For this review, take the finished solid that the model builds, in its own axes (mm). Face numbers are marked on the shaded views. A direction names the side the tool comes from. Coordinates: 2 decimals unless noted, no trailing zeros. Order: outer loops, then holes, each group sorted by start corner. A loop starts at its lowest first (then second) coordinate and runs counter-clockwise, first axis right, second up. Notation, with made-up numbers: M 10.25,-15 L 25.25,-15 A36 ccw 25.25,22 Z; hole C 47.25,-31 d1. An arc over 180 degrees is marked long. Use one line per item in the form item = value. Start each with the question number.
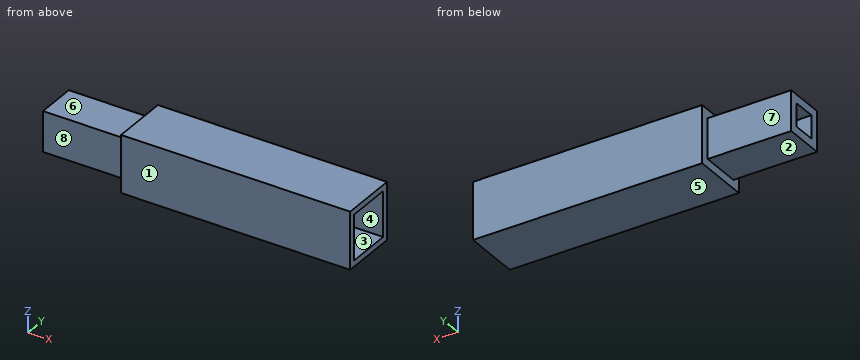
Autodesk Inventor part; units mm, degrees
ref_plane "YZ Plane" through (0, 0, 0) normal (1, 0, 0) x (0, 1, 0)
ref_plane "XZ Plane" through (0, 0, 0) normal (0, 1, 0) x (-1, 0, 0)
ref_plane "XY Plane" through (0, 0, 0) normal (0, 0, 1) x (1, 0, 0)
sketch "Sketch1" plane through (0, 0, 0) normal (1, 0, 0) x (0, 1, 0)
  line L0 (0, 0) -> (25.4, 0)
  line L1 (25.4, 0) -> (25.4, -25.4)
  line L2 (25.4, -25.4) -> (0, -25.4)
  line L3 (0, -25.4) -> (0, 0)
  line L4 (0, 0) -> (3.175, 0)
  line L5 (0, -3.175) -> (0, 0)
  line L6 (3.175, -3.175) -> (22.225, -3.175)
  line L7 (22.225, -3.175) -> (22.225, -22.225)
  line L8 (22.225, -22.225) -> (3.175, -22.225)
  line L9 (3.175, -22.225) -> (3.175, -3.175)
  dimension "d0" = 25.4
  dimension "d1" = 25.4
  dimension "d6" = 19.05
  dimension "d7" = 19.05
extrude "Extrusion1" add sketch "Sketch1" along normal blind 101.6 contours L0 L1 L2 L3 | L6 L7 L8 L9
sketch "Sketch2" plane through (101.6, 0, 0) normal (1, 0, 0) x (0, 0, -1)
  line L0 (22.733, 22.225) -> (22.733, 22.733)
  line L1 (22.733, 22.733) -> (22.225, 22.733)
  line L2 (2.667, 3.175) -> (2.667, 2.667)
  line L3 (2.667, 2.667) -> (3.175, 2.667)
  line L4 (2.667, 2.667) -> (22.733, 2.667)
  line L5 (22.733, 2.667) -> (22.733, 22.733)
  line L6 (22.733, 22.733) -> (2.667, 22.733)
  line L7 (2.667, 22.733) -> (2.667, 2.667)
  point P0 (0, 0)
extrude "Extrusion2" cut sketch "Sketch2" against normal blind 50.8
sketch "Sketch3" plane through (0, 0, 0) normal (-1, 0, 0) x (0, 0, 1)
  line L0 (-25.4, 0) -> (-21.6315, 0)
  line L1 (-21.6315, 3.81) -> (-17.78, 3.81)
  line L2 (-21.6315, 7.62) -> (-21.6315, 3.81)
  line L3 (-3.81, 21.59) -> (-7.62, 21.59)
  line L4 (-3.81, 17.78) -> (-3.81, 21.59)
  line L5 (-21.6315, 3.81) -> (-3.81, 3.81)
  line L6 (-3.81, 3.81) -> (-3.81, 21.59)
  line L7 (-3.81, 21.59) -> (-21.6315, 21.59)
  line L8 (-21.6315, 21.59) -> (-21.6315, 3.81)
  line L9 (-17.8215, 7.6198) -> (-7.62, 7.6198)
  line L10 (-7.62, 7.6198) -> (-7.62, 17.78)
  line L11 (-7.62, 17.78) -> (-17.8215, 17.78)
  line L12 (-17.8215, 17.78) -> (-17.8215, 7.6198)
  point P0 (0, 25.4)
extrude "Extrusion3" add sketch "Sketch3" along normal blind 37.084
properties part number "Right Side PIece Corrected 0.02 inch"
1. The part is to be moulded in two halves that separate along Z. For the marked faces 1, 2, 3 and 4, say which applies: pulls with the +Z half, pulls with the -Z half, needs draft (parallel to the pull), parting line crosses it, or undercut.
2. Tool access review of the marked faces 5, 6, 7 and 8: name each direction out of +Z, -Z, +X, -X, +Y, -Y from which nothing blocks a thin tool from reaching the whole face with its end or side.
3. For pin 1 Ø11 at (x, z) = (-11.5, -15) entering from -Y; pin 2 Ø14 at (x, y) = (-24.5, 15.5) entering from -Z; pin 3 Ø11 at (x, z) = (-27, -15) entering from +Y, all flat-tipped, find the tip position at first contact; note any pin that passes through.
4. To check wall thickness, follow line 1 (Z direction, x = -15.5, y = 9.5); line 2 (Z direction, x = 61, y = 4.5); line 3 (Y direction, x = 66.5, z = -7.5). State the ranges of each line that lie inside material, in increasing order.
5. Consider section B-B, the plane y = 5.5. Write out the cut boundary in (x, z), plus the area to 3 significant figures.
6. Consider section C-C, the plane z = -13.75. Write out the cut boundary in (x, y).
7. Consider section D-D, the plane x = 92. Write out the cut boundary in (y, z).
8. Consider section A-A, the plane x = -22. Write out the cut boundary in (y, z).
Answers follow:
q1.face_1 = needs draft
q1.face_2 = pulls with the -Z half
q1.face_3 = undercut
q1.face_4 = undercut
q2.face_5 = -Z, +X, -X, +Y, -Y
q2.face_6 = +Z, -X, +Y, -Y
q2.face_7 = +Z, -Z, -X, +Y
q2.face_8 = +Z, -Z, -X, -Y
q3.pin_1 = 3.81
q3.pin_2 = -21.63
q3.pin_3 = 21.59
q4.line_1 = -21.63 to -17.82, -7.62 to -3.81
q4.line_2 = -25.4 to -22.73, -2.67 to 0
q4.line_3 = 0 to 2.67, 22.73 to 25.4
q5.outline = M -37.08,-21.63 L 0,-21.63 L 0,-25.4 L 101.6,-25.4 L 101.6,-22.73 L 50.8,-22.73 L 50.8,-2.67 L 101.6,-2.67 L 101.6,0 L 0,0 L 0,-3.81 L -37.08,-3.81 Z
q5.area = 2,220 mm²
q6.outline = M -37.08,3.81 L 0,3.81 L 0,0 L 101.6,0 L 101.6,2.67 L 50.8,2.67 L 50.8,22.73 L 101.6,22.73 L 101.6,25.4 L 0,25.4 L 0,21.59 L -37.08,21.59 L -37.08,17.78 L 0,17.78 L 0,7.62 L -37.08,7.62 Z
q7.outline = M 0,-25.4 L 25.4,-25.4 L 25.4,0 L 0,0 Z; hole M 2.67,-22.73 L 22.73,-22.73 L 22.73,-2.67 L 2.67,-2.67 Z
q8.outline = M 3.81,-21.63 L 21.59,-21.63 L 21.59,-3.81 L 3.81,-3.81 Z; hole M 7.62,-17.82 L 17.78,-17.82 L 17.78,-7.62 L 7.62,-7.62 Z
